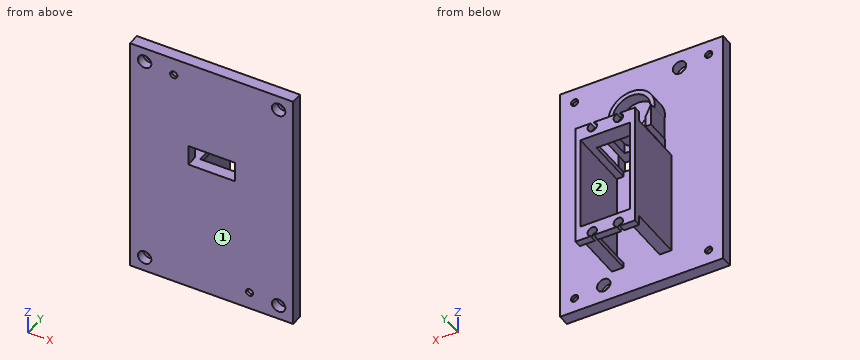
from build123d import *

# Parameters (mm, degrees)
SKETCH1_W           = 71.12
SKETCH1_H           = 106.68
BOSS_EXTRUDE1_DEPTH = 5.08
SKETCH3_W           = 25.908
SKETCH3_H           = 45.7962
SKETCH3_W_2         = 21.59
SKETCH3_H_2         = 41.4782
BOSS_EXTRUDE2_DEPTH = 24.13
SKETCH4_W           = 25.908
SKETCH4_H           = 54.1782
SKETCH4_W_2         = 21.59
SKETCH4_H_2         = 41.4782
BOSS_EXTRUDE3_DEPTH = 3.175
SKETCH5_R           = 2.04968221
CUT_EXTRUDE1_DEPTH  = 3.175
SKETCH7_W           = 15.748
SKETCH7_H           = 20.32
CUT_EXTRUDE3_DEPTH  = 45.7962
SKETCH8_R           = 10.16
BOSS_EXTRUDE4_DEPTH = 7.62
SKETCH9_R           = 8.255
CUT_EXTRUDE4_DEPTH  = 5.08
SKETCH10_W          = 20.32
SKETCH10_H          = 8.89
CUT_EXTRUDE5_DEPTH  = 6.08
SKETCH11_R          = 1.5875
CUT_EXTRUDE6_DEPTH  = 6.08
SKETCH15_R          = 2.921
CUT_EXTRUDE7_DEPTH  = 3.81
SKETCH16_R          = 2.921
CUT_EXTRUDE8_DEPTH  = 3.81
SKETCH17_R          = 1.5875
CUT_EXTRUDE9_DEPTH  = 33.385
BOSS_EXTRUDE5_DEPTH = 10.16


with BuildPart() as part:
    # Sketch1 → Boss-Extrude1 (new body)
    with BuildSketch(Plane(origin=(56.401870569, 0, 2.613156724), x_dir=(1, 0, 0), z_dir=(0, 1, 0))):
        with Locations((-28.531301018, -3.803535099)):
            Rectangle(SKETCH1_W, SKETCH1_H)
    extrude(amount=BOSS_EXTRUDE1_DEPTH)

    # Sketch3 → Boss-Extrude2 (add)
    with BuildSketch(Plane(origin=(56.401870569, 5.08, 2.613156724), x_dir=(1, 0, 0), z_dir=(0, 1, 0))):
        with Locations((-28.531301018, 13.938364901)):
            Rectangle(SKETCH3_W, SKETCH3_H)
        with Locations((-28.531301018, 13.938364901)):
            Rectangle(SKETCH3_W_2, SKETCH3_H_2, mode=Mode.SUBTRACT)
    extrude(amount=BOSS_EXTRUDE2_DEPTH)

    # Sketch4 → Boss-Extrude3 (add)
    with BuildSketch(Plane(origin=(0, 29.21, 0), x_dir=(1, 0, 0), z_dir=(0, 1, 0))):
        with Locations((27.87056955, 11.325208176)):
            Rectangle(SKETCH4_W, SKETCH4_H)
        with Locations((27.87056955, 11.325208176)):
            Rectangle(SKETCH4_W_2, SKETCH4_H_2, mode=Mode.SUBTRACT)
    extrude(amount=BOSS_EXTRUDE3_DEPTH)

    # Sketch5 → Cut-Extrude1 (cut)
    with BuildSketch(Plane(origin=(0, 32.385, 0), x_dir=(1, 0, 0), z_dir=(0, 1, 0))):
        with Locations((22.19366955, 36.471208176)):
            Circle(SKETCH5_R)
        with Locations((33.54746955, 36.471208176)):
            Circle(SKETCH5_R)
        with Locations((22.19366955, -13.820791824)):
            Circle(SKETCH5_R)
        with Locations((33.54746955, -13.820791824)):
            Circle(SKETCH5_R)
    extrude(amount=-CUT_EXTRUDE1_DEPTH, mode=Mode.SUBTRACT)

    # Sketch7 → Cut-Extrude3 (cut)
    with BuildSketch(Plane(origin=(0, 0, -34.223308176), x_dir=(-1, 0, 0), z_dir=(0, 0, -1))):
        with Locations((-27.87056955, 15.24)):
            Rectangle(SKETCH7_W, SKETCH7_H)
    extrude(amount=-CUT_EXTRUDE3_DEPTH, mode=Mode.SUBTRACT)

    # Sketch8 → Boss-Extrude4 (add)
    with BuildSketch(Plane(origin=(0, 5.08, 0), x_dir=(1, 0, 0), z_dir=(0, 1, 0))):
        with Locations((27.87056955, -31.816691824)):
            Circle(SKETCH8_R)
    extrude(amount=BOSS_EXTRUDE4_DEPTH)

    # Sketch9 → Cut-Extrude4 (cut)
    with BuildSketch(Plane(origin=(0, 12.7, 0), x_dir=(1, 0, 0), z_dir=(0, 1, 0))):
        with Locations((27.87056955, -31.816691824)):
            Circle(SKETCH9_R)
    extrude(amount=-CUT_EXTRUDE4_DEPTH, mode=Mode.SUBTRACT)

    # Sketch10 → Cut-Extrude5 (cut, through all)
    with BuildSketch(Plane(origin=(0, 5.08, 0), x_dir=(1, 0, 0), z_dir=(0, 1, 0))):
        with Locations((27.87056955, -16.017891824)):
            Rectangle(SKETCH10_W, SKETCH10_H)
    extrude(amount=-CUT_EXTRUDE5_DEPTH, mode=Mode.SUBTRACT)

    # Sketch11 → Cut-Extrude6 (cut, through all)
    with BuildSketch(Plane(origin=(0, 5.08, 0), x_dir=(1, 0, 0), z_dir=(0, 1, 0))):
        with Locations((44.38056955, 39.303308176)):
            Circle(SKETCH11_R)
        with Locations((11.36056955, -52.136691824)):
            Circle(SKETCH11_R)
    extrude(amount=-CUT_EXTRUDE6_DEPTH, mode=Mode.SUBTRACT)

    # Sketch15 → Cut-Extrude7 (cut)
    with BuildSketch(Plane(origin=(0, 5.08, 0), x_dir=(1, 0, 0), z_dir=(0, 1, 0))):
        with Locations((11.36056955, -52.136691824)):
            Circle(SKETCH15_R)
        with Locations((44.38056955, 39.303308176)):
            Circle(SKETCH15_R)
    extrude(amount=-CUT_EXTRUDE7_DEPTH, mode=Mode.SUBTRACT)

    # Sketch16 → Cut-Extrude8 (cut)
    with BuildSketch(Plane.XZ):
        with Locations((-1.33943045, 53.406691824)):
            Circle(SKETCH16_R)
        with Locations((57.08056955, 53.406691824)):
            Circle(SKETCH16_R)
        with Locations((57.08056955, -40.573308176)):
            Circle(SKETCH16_R)
        with Locations((-1.33943045, -40.573308176)):
            Circle(SKETCH16_R)
    extrude(amount=-CUT_EXTRUDE8_DEPTH, mode=Mode.SUBTRACT)

    # Sketch17 → Cut-Extrude9 (cut, through all)
    with BuildSketch(Plane.XZ):
        with Locations((-1.33943045, 53.406691824)):
            Circle(SKETCH17_R)
        with Locations((57.08056955, 53.406691824)):
            Circle(SKETCH17_R)
        with Locations((57.08056955, -40.573308176)):
            Circle(SKETCH17_R)
        with Locations((-1.33943045, -40.573308176)):
            Circle(SKETCH17_R)
    extrude(amount=-CUT_EXTRUDE9_DEPTH, mode=Mode.SUBTRACT)

    # Sketch23 → Boss-Extrude5 (add)
    with BuildSketch(Plane(origin=(0, 5.08, 0), x_dir=(1, 0, 0), z_dir=(0, 1, 0))):
        Polygon((20.37756955, -20.462891824), (17.83756955, -20.462891824), (17.83756955, -30.215282757), (20.37756955, -24.955164953), align=None)
        Polygon((35.36356955, -20.462891824), (37.90356955, -20.462891824), (37.90356955, -30.215282757), (35.36356955, -24.955164953), align=None)
    extrude(amount=BOSS_EXTRUDE5_DEPTH)


solid = part.part
Geometry check sheet. Reference: the model listing, model coordinates, mm. Face numbers are marked on the shaded views. Round coordinates to 2 decimals unless told otherwise and drop trailing zeros. Order: outer loops, then holes, each group sorted by start corner. A loop starts at its lowest first (then second) coordinate and runs counter-clockwise, first axis right, second up. Notation, with made-up numbers: M -12.5,14.5 L -2.5,14.5 A17 cw -2.5,47.5 Z; hole C -7.75,17 d6. An arc over 180 degrees is marked long. Write each question's results on one line, items separated by ' | '. Start each with the question number.
1. Cross-section at D-D on z = -3.5. Record the boundary of the cut face in (x, y) (3 decimals), plus the area to 3 significant figures.
2. Cross-section at A-A on y = 27.5. Record the boundary of the cut face in (x, z), plus the area to 3 significant figures.
3. Material ranges on L1, parallel to X at y = 29.5, z = -19; L2, parallel to Z at x = -1, y = 5; L3, parallel to X at y = 16.5, z = 11, recorded low to high. Write a range as from..to.
4. Go/stop test with flat-tipped pins: P1, Ø1.7, axis at y = 11, z = 10, coming from the +X side; P2, Ø1, axis at x = 38, y = 30, coming from the -Z side; P3, Ø8, axis at x = 49.5, z = 42.5, coming from the +Y side; P4, Ø10, axis at x = 11, y = 10, coming from the -Z side. Record where each tip stops, or that it passes through.
5. Cross-section at B-B on y = 21. Record the boundary of the cut face in (x, z).
6. Draft check along Z on the marked faces 1 and 2. Enter one of: pulls with the +Z half, pulls with the -Z half, needs draft (parallel to the pull), parting line crosses it, or undercut.
7. Cross-section at C-C on x = 30. Record the boundary of the cut face in (y, z) (3 decimals).
Resolved:
1) outline: M -7.689,0 L 63.431,0 L 63.431,5.08 L 40.825,5.08 L 40.825,32.385 L 38.666,32.385 L 38.666,5.08 L 17.076,5.08 L 17.076,32.385 L 14.917,32.385 L 14.917,5.08 L -7.689,5.08 Z | area: 479 mm2
2) outline: M 14.92,-34.22 L 40.82,-34.22 L 40.82,11.57 L 14.92,11.57 Z; hole M 17.08,-32.06 L 38.67,-32.06 L 38.67,9.41 L 17.08,9.41 Z | area: 291 mm2
3) L1: 14.92..17.08, 38.67..40.82 | L2: -46.92..-42.12, -39.02..51.86, 54.96..59.76 | L3: 14.92..20, 35.74..40.82
4) P1: x = 40.82 | P2: z = -38.41 | P3: y = 5.08 | P4: z = -46.92
5) outline: M 14.92,-34.22 L 20,-34.22 L 20,-32.06 L 17.08,-32.06 L 17.08,9.41 L 20,9.41 L 20,11.57 L 14.92,11.57 Z; M 35.74,-34.22 L 40.82,-34.22 L 40.82,11.57 L 35.74,11.57 L 35.74,9.41 L 38.67,9.41 L 38.67,-32.06 L 35.74,-32.06 Z
6) face 1: needs draft | face 2: undercut
7) outline: M 0,-46.923 L 5.08,-46.923 L 5.08,11.573 L 0,11.573 Z; M 0,20.463 L 5.08,20.463 L 5.08,21.882 L 12.7,21.882 L 12.7,23.841 L 7.62,23.841 L 7.62,39.792 L 12.7,39.792 L 12.7,41.751 L 5.08,41.751 L 5.08,59.757 L 0,59.757 Z; M 25.4,-34.223 L 29.21,-34.223 L 29.21,-38.414 L 32.385,-38.414 L 32.385,-32.064 L 25.4,-32.064 Z; M 25.4,9.414 L 32.385,9.414 L 32.385,15.764 L 29.21,15.764 L 29.21,11.573 L 25.4,11.573 Z
